Check sheet for the modelled part. Datum: model origin and axes. Units: mm. A direction names the side the tool comes from. Round coordinates to 2 decimals unless told otherwise and drop trailing zeros. Order: outer loops, then holes, each group sorted by start corner. A loop starts at its lowest first (then second) coordinate and runs counter-clockwise, first axis right, second up.
Q1. Scan lines: probe 1 along Y at (x, z) = (124, 184); probe 2 along Z at (x, y) = (232.5, -41); probe 3 along Y at (x, z) = (1076.5, 125). Record each from-to range of solid material in increasing order.
Q2. Cross-section at C-C on y = -69. Record the cut outline in (x, z), then the cut area to 3 significant figures.
Q3. Depth check by flat-ended pin: P1, Ø4, axis at x = 354, y = -182, coming from the +Z side; P2, Ø5, axis at y = -56, z = 80, coming from the +X side. Enter the tip coordinate at first touch or a pass-through.
Q4. Cross-section at A-A on z = 296. Record the cut outline in (x, y), then the cut area to 3 significant figures.
Q5. Mould release check, pull along Y, two halves, no side actions. Record for faces 4 (the flat face through (1130.2, -4.8, 216)), 5 (the flat face through (300, -68, 106)), 6 (the flat face through (433, -150, 0)): +Y half, -Y half, draft (parallel to the pull), parting line (faces both ways), or undercut.
Q6. Set-up check for faces 1 (the flat face through (557, -5, 220)), 2 (the flat face through (417, -290, 215)), 3 (the flat face through (305, -68, 106)): record each of +Z, -Z, +X, -X, +Y, -Y from which the full face is reachable in a straight line by a thin tool's end or side.
Q7. Cross-section at B-B on x = 248. Record the cut outline in (y, z), then the cut area to 3 significant figures.
Q8. Cross-section at D-D on z = 158. Record the cut outline in (x, y).
from build123d import *

# Parameters (mm, degrees)
F1_DEPTH = 1200
F4_DEPTH = 5
F5_W     = 1200
F5_H     = 230
F6_DEPTH = 4
F7_R     = 2
F9_DEPTH = 430.001


# Not quite as in the source:
# - a feature names something its author has since deleted; it is built from what else it names


with BuildPart() as f1:
    # F0 (on Right) → F1 (new body)
    with BuildSketch(Plane.YZ):
        Polygon((-295, 0), (0, 0), (0, 430), (-5, 430), (-5, 5), (-290, 5), (-290, 430), (-295, 430), align=None)
    extrude(amount=F1_DEPTH)



with BuildPart() as f4:
    # F3 (on offset) → F4 (new body)
    with BuildSketch(Plane.YZ.offset(300)):
        Polygon((-230, 0), (-5, 0), (-5, 360), align=None)
    extrude(amount=F4_DEPTH)


with BuildPart() as f1_1:
    add(f1.part)

    add(f4.part)  # F6 merges F4
    # F5 (on Top) → F6 (join)
    with BuildSketch(Plane.XY):
        with Locations((600, -115)):
            Rectangle(F5_W, F5_H)
    extrude(amount=F6_DEPTH)

    # F7
    f7_edges = [f1_1.edges().sort_by_distance(p)[0] for p in [
        (600, 0, 0),
        (600, -295, 0),
    ]]
    fillet(f7_edges, radius=F7_R)

    # F8 (on face) → F9 (cut, through all)
    with BuildSketch(Plane.XY.offset(430)):
        Polygon((1135, 0), (840, -295), (1200, -295), (1200, 0), align=None)
    extrude(amount=-F9_DEPTH, mode=Mode.SUBTRACT)


solid = f1_1.part
Results found:
1. probe 1: y = -295 to -290, -5 to 0
1. probe 2: z = 0 to 5
1. probe 3: y = -5 to 0
2. outline: (0, 0) - (1066, 0) - (1066, 5) - (305, 5) - (305, 257.6) - (300, 257.6) - (300, 5) - (0, 5) - close
2. area: 6,590 mm2
3. P1: stops at z = 5
3. P2: stops at x = 305
4. outline: (0, -295) - (840, -295) - (845, -290) - (0, -290) - close; (0, -5) - (300, -5) - (300, -45) - (305, -45) - (305, -5) - (1130, -5) - (1135, 0) - (0, 0) - close
4. area: 10,100 mm2
5. face 4: -Y half
5. face 5: undercut
5. face 6: draft
6. face 1: +Z
6. face 2: +Z, +X, -X
6. face 3: +Z, +X
7. outline: (-295, 2) arc R2 ccw to (-293, 0) - (-2, 0) arc R2 ccw to (0, 2) - (0, 430) - (-5, 430) - (-5, 5) - (-290, 5) - (-290, 430) - (-295, 430) - close
7. area: 5,720 mm2
8. outline: (0, -295) - (840, -295) - (845, -290) - (0, -290) - close; (0, -5) - (300, -5) - (300, -131.25) - (305, -131.25) - (305, -5) - (1130, -5) - (1135, 0) - (0, 0) - close
